Build history of the part. All positions in model axes, mm. Give positions to 0.01 mm unless a question says otherwise; leave off trailing zeros. Order: outer loops, then holes, each group sorted by start corner. A loop starts at its lowest first (then second) coordinate and runs counter-clockwise, first axis right, second up. Notation, with made-up numbers: (-1.5, -29.75) - (55.5, -29.75) arc R25 cw to (55.5, 6.25) - close; hole circle Ø5 at (-37.5, 75). An arc over 180 degrees is marked (long way). Answer in a Markdown table with one row per item.
```python
from build123d import *

# Parameters (mm, degrees)
SKETCH1_W           = 46
SKETCH1_H           = 50
BOSS_EXTRUDE1_DEPTH = 3
SKETCH2_W           = 3
SKETCH2_H           = 15
CUT_EXTRUDE1_DEPTH  = 53.999062732
LPATTERN1_COUNT     = 3
LPATTERN1_PITCH     = 22.8
SKETCH3_W           = 7.8
SKETCH3_H           = 3
BOSS_EXTRUDE2_DEPTH = 3
LPATTERN2_COUNT     = 2
LPATTERN2_PITCH     = 22.8


with BuildPart() as part:
    # Sketch1 → Boss-Extrude1 (new body)
    with BuildSketch(Plane.XY):
        with Locations((-17.993460648, -8.457986111)):
            Rectangle(SKETCH1_W, SKETCH1_H)
    extrude(amount=BOSS_EXTRUDE1_DEPTH)

    # Sketch2 → Cut-Extrude1 (cut, through all)
    with BuildSketch(Plane.XY.offset(3)):
        with Locations((-39.493460648, 1.242013889)):
            Rectangle(SKETCH2_W, SKETCH2_H)
        with Locations((3.506539352, 1.242013889)):
            Rectangle(SKETCH2_W, SKETCH2_H)
    cut_extrude1 = extrude(amount=-CUT_EXTRUDE1_DEPTH, mode=Mode.SUBTRACT)

    # LPattern1: Cut-Extrude1 ×3
    with Locations(*[(0, -i * LPATTERN1_PITCH, 0) for i in range(1, LPATTERN1_COUNT)]):
        add(cut_extrude1, mode=Mode.SUBTRACT)

    # Sketch3 → Boss-Extrude2 (add)
    with BuildSketch(Plane(origin=(0, 16.542013889, 0), x_dir=(1, 0, 0), z_dir=(0, 1, 0))):
        with Locations((-29.393460648, -1.5)):
            Rectangle(SKETCH3_W, SKETCH3_H)
    boss_extrude2 = extrude(amount=BOSS_EXTRUDE2_DEPTH)

    # LPattern2: Boss-Extrude2 ×2
    with Locations(*[(i * LPATTERN2_PITCH, 0, 0) for i in range(1, LPATTERN2_COUNT)]):
        add(boss_extrude2)


solid = part.part
```
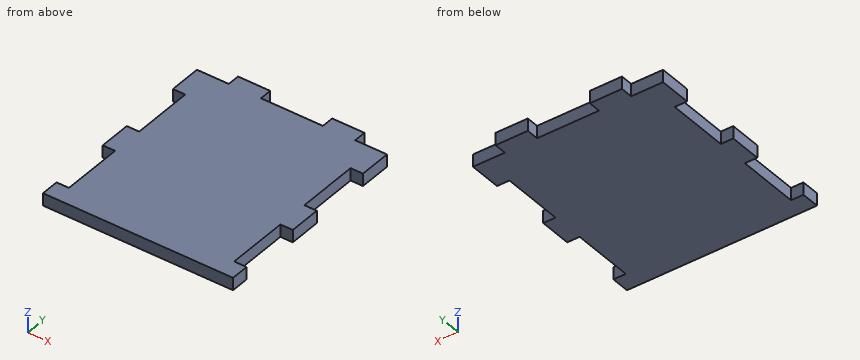
1. Cut at A-A on z = 1.2. Write the cut outline in (x, y), and give its area (3 significant figures).
Check result:
| item | result |
|---|---|
| outline | (-40.99, -33.46) - (5.01, -33.46) - (5.01, -29.06) - (2.01, -29.06) - (2.01, -14.06) - (5.01, -14.06) - (5.01, -6.26) - (2.01, -6.26) - (2.01, 8.74) - (5.01, 8.74) - (5.01, 16.54) - (-2.69, 16.54) - (-2.69, 19.54) - (-10.49, 19.54) - (-10.49, 16.54) - (-25.49, 16.54) - (-25.49, 19.54) - (-33.29, 19.54) - (-33.29, 16.54) - (-40.99, 16.54) - (-40.99, 8.74) - (-37.99, 8.74) - (-37.99, -6.26) - (-40.99, -6.26) - (-40.99, -14.06) - (-37.99, -14.06) - (-37.99, -29.06) - (-40.99, -29.06) - close |
| area | 2,170 mm² |
2. Cut at B-B on y = 0. Write the cut outline in (x, z).
Check result:
| item | result |
|---|---|
| outline | (-37.99, 0) - (2.01, 0) - (2.01, 3) - (-37.99, 3) - close |
3. Cut at C-C on x = -17.5. Write the cut outline in (y, z).
Check result:
| item | result |
|---|---|
| outline | (-33.46, 0) - (16.54, 0) - (16.54, 3) - (-33.46, 3) - close |
4. Probe line 1 (X direction, y = -23.5, z = 2.4); line 2 (Y direction, x = -1, z = 2.15). List the from-to ranges inside material, lowest first.
Check result:
| item | result |
|---|---|
| line 1 | x = -37.99 to 2.01 |
| line 2 | y = -33.46 to 16.54 |
5. Drop flat-ended pins along their axis: P1, Ø1.5, axis at y = -24.5, z = 2, coming from the -X side; P2, Ø1.5, axis at x = -1, z = 1.5, coming from the +Y side; P3, Ø1.5, axis at y = -23.5, z = 2, coming from the +X side; P4, Ø12, axis at x = -15, y = -27.5, coming from the -Z side. Give the stop position or say it passes through.
Check result:
| item | result |
|---|---|
| P1 | stops at x = -37.99 |
| P2 | stops at y = 16.54 |
| P3 | stops at x = 2.01 |
| P4 | stops at z = 0 |
